Geometry: see drawing. Coordinates: mm, zero at the bounding-box minimum. Give positions to 0.01 mm unless a question says otherwise; leave off trailing zeros. Write each loop counter-clockwise with the first axis right and the second up, starting at its lowest first coordinate (ties: lowest second). Pieces come first, ordered by that corner, then holes. Notation, with made-up numbers: (-16, 50.5) - (4, 50.5) arc R10 cw to (4, 59.5) - close; hole circle Ø3 at (1, 6.25). An arc over 180 degrees is marked (long way). One line per question, with ' | ' between items. Start each with the question number.
(1) Pin query (flat end, axial travel): pin 1 (6 mm diameter, centred on y = 159.5, z = 15, fed in from -X). Return the tip coordinate at first contact, or that it passes through.
(2) Section B-B, the plane y = 170.5. Return loops of the section in (x, z) (3 decimals).
(3) Ray query, line 1 (Y direction, x = 25.4, z = 22.9); line 2 (Z direction, x = 17, y = 90) (3 decimals); line 3 (X direction, y = 95.5, z = 3.5) (3 decimals). Return the intervals inside material, ascending. Write a range as [from, to].
(4) Section C-C, the plane z = 12. Return loops of the section in (x, y) (3 decimals), plus the area to 3 significant figures.
(5) Section A-A, the plane x = 25.4. State how many separate pieces and enclosed holes the cut face has, plus the area to 3 significant figures.
(6) Section D-D, the plane y = 114.3. Return loops of the section in (x, z) (1 decimal).
(7) Draft query along Z for the marked faces 1, 2, 3 and 4. Return one class per face: +Z half, -Z half, draft (parallel to the pull), parting line (faces both ways), or undercut.
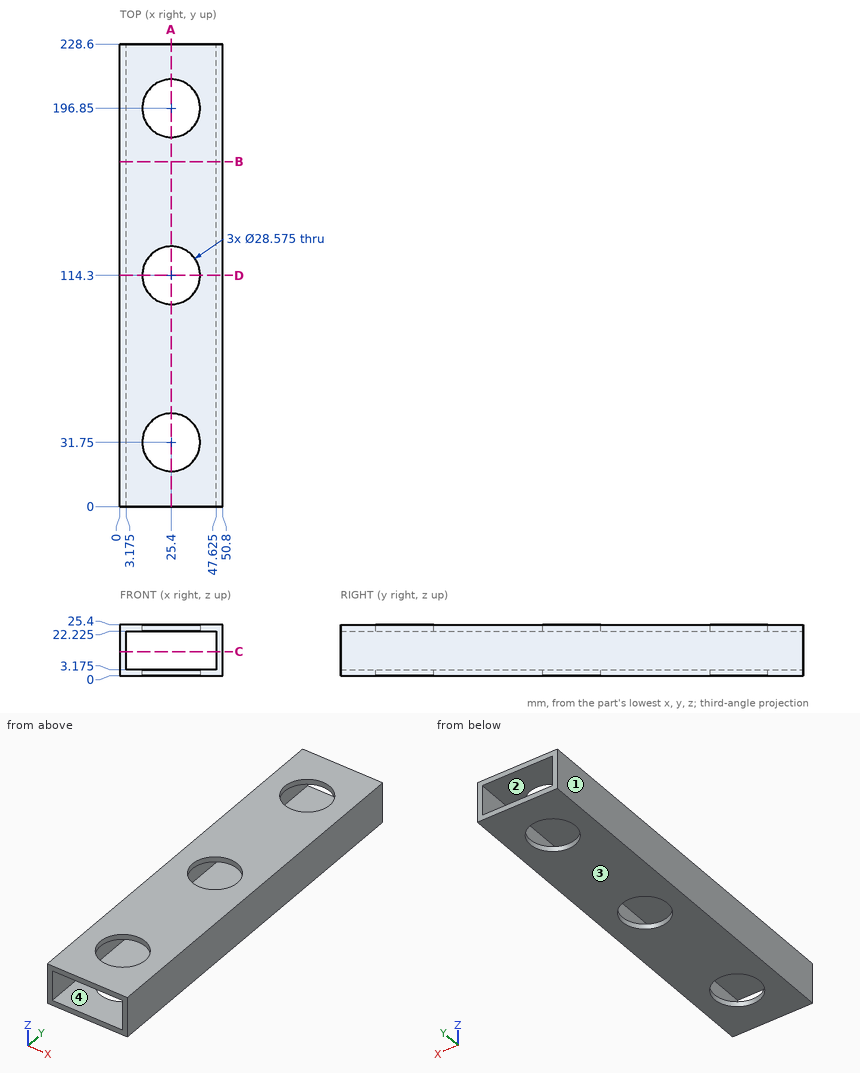
Check sheet entries:
1) pin 1: x = 0
2) outline: (0, 0) - (50.8, 0) - (50.8, 25.4) - (0, 25.4) - close; hole (3.175, 3.175) - (47.625, 3.175) - (47.625, 22.225) - (3.175, 22.225) - close
3) line 1: [0, 17.46], [46.04, 100.01], [128.59, 182.56], [211.14, 228.6] | line 2: [0, 3.175], [22.225, 25.4] | line 3: [0, 3.175], [47.625, 50.8]
4) outline: (0, 0) - (3.175, 0) - (3.175, 228.6) - (0, 228.6) - close; (47.625, 0) - (50.8, 0) - (50.8, 228.6) - (47.625, 228.6) - close | area: 1,450 mm²
5) separate pieces: 8 | enclosed holes: 0 | area: 907 mm²
6) outline: (0, 0) - (11.1, 0) - (11.1, 3.2) - (3.2, 3.2) - (3.2, 22.2) - (11.1, 22.2) - (11.1, 25.4) - (0, 25.4) - close; (39.7, 0) - (50.8, 0) - (50.8, 25.4) - (39.7, 25.4) - (39.7, 22.2) - (47.6, 22.2) - (47.6, 3.2) - (39.7, 3.2) - close
7) face 1: draft | face 2: undercut | face 3: -Z half | face 4: undercut
